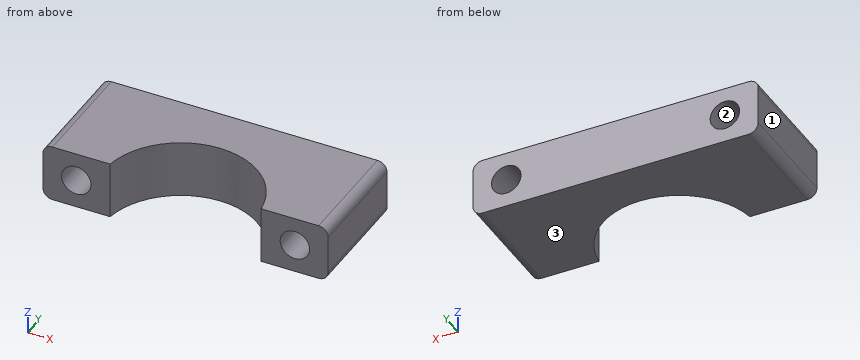
from build123d import *

# Parameters (mm, degrees)
SKETCH1_W           = 30
SKETCH1_H           = 12
BOSS_EXTRUDE1_DEPTH = 6
SKETCH2_R           = 8
CUT_EXTRUDE1_DEPTH  = 18.23368794
SKETCH3_R           = 1.55
CUT_EXTRUDE2_DEPTH  = 21.124611797
FILLET1_R           = 1


with BuildPart() as part:
    # Sketch1 → Boss-Extrude1 (new body)
    with BuildSketch(Plane.XY):
        Rectangle(SKETCH1_W, SKETCH1_H)
    extrude(amount=BOSS_EXTRUDE1_DEPTH)

    # Sketch2 → Cut-Extrude1 (cut, through all)
    with BuildSketch(Plane.XY.offset(6)):
        with Locations((0, -7)):
            Circle(SKETCH2_R)
    extrude(amount=-CUT_EXTRUDE1_DEPTH, mode=Mode.SUBTRACT)

    # Sketch3 → Cut-Extrude2 (cut, through all)
    with BuildSketch(Plane(origin=(0, 6, 0), x_dir=(1, 0, 0), z_dir=(0, 1, 0))):
        with Locations(Location((-11.5, -3, 0), (0, 0, 270))):
            Circle(SKETCH3_R)
        with Locations(Location((11.5, -3, 0), (0, 0, 270))):
            Circle(SKETCH3_R)
    extrude(amount=-CUT_EXTRUDE2_DEPTH, mode=Mode.SUBTRACT)

    # Fillet1
    fillet1_edges = [part.edges().sort_by_distance(p)[0] for p in [
        (-15, 0, 6),
        (15, 0, 6),
        (-15, 0, 0),
        (15, 0, 0),
    ]]
    fillet(fillet1_edges, radius=FILLET1_R)


solid = part.part
CAD build for the part. Positions are in the model's coordinates, mm. Face numbers are marked on the shaded views. Round coordinates to 2 decimals unless told otherwise and drop trailing zeros. Write each loop counter-clockwise with the first axis right and the second up, starting at its lowest first coordinate (ties: lowest second). Pieces come first, ordered by that corner, then holes. Notation, with made-up numbers: (1.5, 2) -> (41.5, 2) arc R23 cw to (41.5, 37) -> close; hole circle Ø10 at (82.5, 88). An arc over 180 degrees is marked (long way). Answer as a JSON object with one key per item and string values.
(1) Two-plate mould, pull along Z, no slides. Class the marked faces 1, 2 and 3: +Z half, -Z half, draft (parallel to the pull), parting line (faces both ways), or undercut.
Reported:
{"face 1": "draft", "face 2": "undercut", "face 3": "-Z half"}
(2) Band-saw the part on C-C, the plane z = 3. List the corners of the cut face in (x, y), then the cut area to 3 significant figures.
Reported:
{"outline": "(-15, -6) -> (-13.05, -6) -> (-13.05, 6) -> (-15, 6) -> close; (-9.95, -6) -> (-7.94, -6) arc R8 cw to (7.94, -6) -> (9.95, -6) -> (9.95, 6) -> (-9.95, 6) -> close; (13.05, -6) -> (15, -6) -> (15, 6) -> (13.05, 6) -> close", "area": "201 mm^2"}
(3) Probe probe 1 along X at (y, z) = (1.75, 3); probe 2 along X at (y, z) = (0.25, 3); probe 3 along X at (y, z) = (3, 1.8). List the from-to ranges inside material, lowest first. Write a range as [from, to].
Reported:
{"probe 1": "x = [-15, -13.05], [-9.95, 9.95], [13.05, 15]", "probe 2": "x = [-15, -13.05], [-9.95, -3.38], [3.38, 9.95], [13.05, 15]", "probe 3": "x = [-15, -12.48], [-10.52, 10.52], [12.48, 15]"}
(4) Band-saw the part on D-D, the plane y = 5.25. List the corners of the cut face in (x, z).
Reported:
{"outline": "(-15, 1) arc R1 ccw to (-14, 0) -> (14, 0) arc R1 ccw to (15, 1) -> (15, 5) arc R1 ccw to (14, 6) -> (-14, 6) arc R1 ccw to (-15, 5) -> close; hole circle Ø3.1 at (-11.5, 3); hole circle Ø3.1 at (11.5, 3)"}
(5) Band-saw the part on A-A, the plane x = 11.5. List the corners of the cut face in (y, z), then the cut area to 3 significant figures.
Reported:
{"outline": "(-6, 0) -> (6, 0) -> (6, 1.45) -> (-6, 1.45) -> close; (-6, 4.55) -> (6, 4.55) -> (6, 6) -> (-6, 6) -> close", "area": "34.8 mm^2"}
(6) Band-saw the part on B-B, the plane y = -3.5. List the corners of the cut face in (x, z).
Reported:
{"outline": "(-15, 1) arc R1 ccw to (-14, 0) -> (-7.19, 0) -> (-7.19, 6) -> (-14, 6) arc R1 ccw to (-15, 5) -> close; (7.19, 0) -> (14, 0) arc R1 ccw to (15, 1) -> (15, 5) arc R1 ccw to (14, 6) -> (7.19, 6) -> close; hole circle Ø3.1 at (-11.5, 3); hole circle Ø3.1 at (11.5, 3)"}
